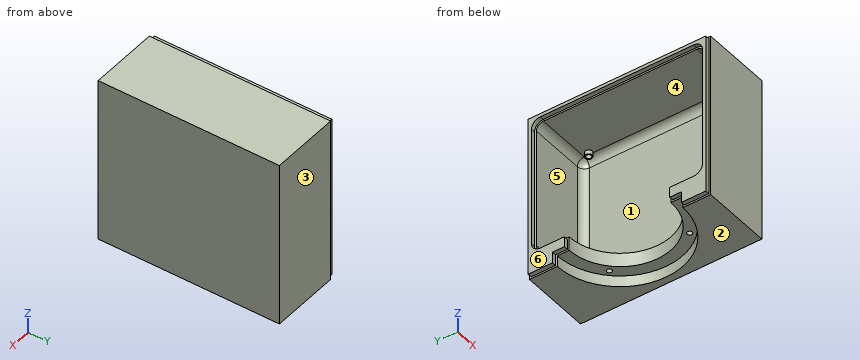
Autodesk Inventor part; units mm, degrees
ref_plane "Work Plane1" through (-95, 0, -119) normal (-1, 0, 0) x (0, 0, 1)
ref_plane "Work Plane2" through (-50, 0, -119) normal (-1, 0, 0) x (0, 0, 1)
ref_plane "YZ Plane" through (0, 0, 0) normal (1, 0, 0) x (0, 1, 0)
sketch "Sketch1" plane through (0, 0, 0) normal (0, 1, 0) x (-1, 0, 0)
  line L0 (0, 0) -> (100, 0)
  line L1 (100, 0) -> (100, -119)
  line L2 (100, -119) -> (0, -119)
  line L3 (0, -119) -> (0, 0)
  dimension "d0" = 119
  dimension "d1" = 100
extrude "Extrusion1" add sketch "Sketch1" along normal blind 130
sketch "Sketch2" plane through (0, 0, -119) normal (0, 0, -1) x (-1, 0, 0)
  circle A0 centre (50, 65) radius 45
  line L0 (100, 0) -> (100, 130)
  line L1 (0, 0) -> (0, 130)
  line L2 (0, 0) -> (100, 0)
  line L3 (0, 130) -> (100, 130)
  circle A1 centre (50, 65) radius 36.5
  circle A2 centre (28.0236, 99.1226) radius 1.9
  line L4 (25.6342, 102.8326) -> (74.3658, 27.1674) construction
  line L5 (12.1674, 40.6342) -> (87.8326, 89.3658) construction
  dimension "d6" = 90
  dimension "d7" = 100
  dimension "d8" = 50
  dimension "d9" = 65
  dimension "d10" = 130
  dimension "d11" = 73
  dimension "d12" = 3.8
extrude "Extrusion2" cut sketch "Sketch2" against normal blind 8 contours A0 | A1 | A2
extrude "Extrusion3" cut sketch "Sketch2" against normal blind 18 contours A1
ref_plane "Work Plane1" through (-95, 0, -119) normal (-1, 0, 0) x (0, 0, 1)
sketch "Sketch3" plane through (-95, 0, -119) normal (-1, 0, 0) x (0, 0, 1)
  line L0 (18, 28.5) -> (18, 101.5)
  line L1 (119, 130) -> (119, 0)
  line L2 (119, 0) -> (0, 0)
  line L3 (0, 0) -> (0, 65)
  line L4 (8, 65) -> (0, 65)
  line L5 (0, 130) -> (119, 130)
  line L6 (0, 65) -> (0, 130)
  line L7 (114, 125) -> (18, 125)
  line L8 (18, 125) -> (18, 5)
  line L9 (18, 5) -> (114, 5)
  line L10 (114, 5) -> (114, 125)
  dimension "d16" = 5
  dimension "d17" = 5
  dimension "d18" = 5
extrude "Extrusion4" cut sketch "Sketch3" against normal blind 90 and the other way blind 90 contours L0 L8 L7 L10 L9
fillet "Fillet1" radius 5 8 edges at (-52.5, 5, -5) (-5, 5, -53) (-5, 65, -5) (-5, 125, -53) (-52.5, 125, -5) (-52.5, 5, -101) (-52.5, 125, -101) (-5, 65, -101)
sketch "Sketch8" plane through (-100, 0, -119) normal (-1, 0, 0) x (0, 0, 1)
  point P0 (119, 0)
sketch "Sketch10" plane through (-100, 0, -119) normal (-1, 0, 0) x (0, 0, 1)
  line L0 (0, 0) -> (119, 0)
  line L1 (119, 0) -> (119, 130)
  line L2 (0, 130) -> (119, 130)
  line L3 (0, 0) -> (0, 130)
extrude "Extrusion10" add sketch "Sketch10" along normal blind 5
sketch "Sketch12" plane through (0, 130, 0) normal (0, 1, 0) x (1, 0, 0)
  line L0 (0, 119) -> (-105, 119)
  line L1 (-105, 0) -> (-105, 119)
  line L2 (0, 0) -> (-105, 0)
  line L3 (0, 0) -> (0, 119)
  line L4 (-105, 0) -> (-100, 0)
  line L5 (-100, 0) -> (-100, 119)
  line L6 (-100, 119) -> (-105, 119)
  line L7 (-105, 119) -> (-105, 0)
  line L8 (-100, 20) -> (-105, 25)
  line L9 (-105, 40) -> (-100, 45)
  line L10 (-105, 94) -> (-100, 99)
  line L11 (-100, 74) -> (-105, 79)
  dimension "d82" = 119
  dimension "d86" = 5
  dimension "d87" = 45
  dimension "d88" = 45
  dimension "d90" = 45
  dimension "d91" = 45
  dimension "d92" = 20
  dimension "d93" = 25
  dimension "d94" = 20
  dimension "d95" = 25
extrude "Extrusion11" cut sketch "Sketch12" against normal blind 127 contours L5 L11 L1 L10 | L8 L1 L9 L5
fillet "Fillet2" radius 1 8 edges at (-105, 66.5, -25) (-100, 127.5, -20) (-105, 66.5, -40) (-100, 127.5, -45) (-105, 66.5, -79) (-100, 127.5, -74) (-105, 66.5, -94) (-100, 127, -99)
sketch "Sketch13" plane through (-10, 120, -5) normal (0, 0, -1) x (-1, 0, 0)
  line L0 (82.5, 0) -> (-2.5, 0)
  line L1 (-2.5, 0) -> (-2.5, -110)
  line L2 (-2.5, -110) -> (82.5, -110)
  line L3 (82.5, -110) -> (82.5, 0)
  line L4 (-5, 0) -> (-5, -110)
  line L5 (85, -110) -> (85, 0)
  circle A0 centre (78.5, -4.3) radius 1.8
  circle A1 centre (78.5, -4.3) radius 2.5
  line L6 (78.5, -4.3) -> (78.5, -140.0823) construction
  line L7 (78.5, -4.3) -> (-34.9987, -4.3) construction
  line L8 (1.5, 27.6777) -> (1.5, -220.2724) construction
  line L9 (-45.8754, -105.7) -> (99.6232, -105.7) construction
  line L10 (80, 5) -> (0, 5) construction
  line L11 (0, -115) -> (80, -115) construction
  circle A2 centre (78.5, -105.7) radius 1.8
  circle A3 centre (78.5, -105.7) radius 2.5
  circle A4 centre (1.5, -105.7) radius 1.8
  circle A5 centre (1.5, -105.7) radius 2.5
  circle A6 centre (1.5, -4.3) radius 1.8
  circle A7 centre (1.5, -4.3) radius 2.5
  point P0 (-10, -120)
  dimension "d97" = 85
  dimension "d98" = 110
  dimension "d99" = 90
  dimension "d100" = 2.5
  dimension "d101" = 4
  dimension "d102" = 4.3
  dimension "d103" = 3.6
  dimension "d104" = 5
  dimension "d105" = 4.3
  dimension "d107" = 120
  dimension "d108" = 5
  dimension "d109" = 4
  dimension "d110" = 3.6
  dimension "d111" = 5
  dimension "d112" = 3.6
  dimension "d113" = 5
  dimension "d114" = 3.6
  dimension "d115" = 5
extrude "Extrusion12" add sketch "Sketch13" along normal blind 3 contours A1 | A3 | A5 | A7
sketch "Sketch14" plane through (-105, 0, -119) normal (-1, 0, 0) x (0, 0, 1)
  line L0 (19.5, 52) -> (19.5, 34) construction
  line L1 (18, 52) -> (18, 34)
  line L2 (21, 34) -> (21, 52)
  arc A0 (21, 52) -> (18, 52) centre (19.5, 52) ccw
  arc A1 (18, 34) -> (21, 34) centre (19.5, 34) ccw
  line L3 (0, 130) -> (0, 0)
  line L4 (0, 0) -> (119, 0)
  point P0 (19.5, 43)
  dimension "d118" = 18
  dimension "d119" = 3
  dimension "d121" = 18
  dimension "d122" = 34
extrude "Extrusion13" cut sketch "Sketch14" against normal blind 20
sketch "Sketch15" plane through (-50, 65, -111) normal (0, 0, -1) x (-1, 0, 0)
  circle A0 centre (0, 0) radius 45 construction
  line L0 (31.8198, 31.8198) -> (-31.8198, -31.8198) construction
  line L1 (31.8198, -31.8198) -> (-31.8198, 31.8198) construction
  circle A1 centre (0, 0) radius 36.5 construction
  circle A2 centre (0, 0) radius 40.75 construction
  line L2 (0, -45) -> (0, 45) construction
  line L3 (-40, -60) -> (40, -60) construction
  circle A3 centre (28.8146, 28.8146) radius 1.8
  circle A4 centre (-28.8146, 28.8146) radius 1.8
  circle A5 centre (28.8146, -28.8146) radius 1.8
  circle A6 centre (-28.8146, -28.8146) radius 1.8
  point P0 (-50, -65)
  dimension "d125" = 45
  dimension "d126" = 73
  dimension "d129" = 90
  dimension "d130" = 4.25
  dimension "d131" = 3.6
  dimension "d135" = 3.6
  dimension "d136" = 3.6
  dimension "d137" = 3.6
extrude "Extrusion14" cut sketch "Sketch15" against normal blind 40
ref_plane "Work Plane2" through (-50, 0, -119) normal (-1, 0, 0) x (0, 0, 1)
split "Split1" plane through (-50, 0, -119) removes the side toward (-1, 0, 0)
sketch "Sketch18" plane through (-50, 0, -119) normal (-1, 0, 0) x (0, 0, 1)
  line L0 (8, 110) -> (0, 110)
  line L1 (8, 101.5) -> (8, 110)
  line L2 (18, 101.5) -> (8, 101.5)
  line L3 (18, 120) -> (18, 101.5)
  arc A0 (23, 125) -> (18, 120) centre (23, 120) ccw
  line L4 (109, 125) -> (23, 125)
  arc A1 (114, 120) -> (109, 125) centre (109, 120) ccw
  line L5 (114, 10) -> (114, 120)
  arc A2 (109, 5) -> (114, 10) centre (109, 10) ccw
  line L6 (23, 5) -> (109, 5)
  arc A3 (18, 10) -> (23, 5) centre (23, 10) ccw
  line L7 (18, 28.5) -> (18, 10)
  line L8 (8, 28.5) -> (18, 28.5)
  line L9 (8, 20) -> (8, 28.5)
  line L10 (0, 20) -> (8, 20)
  line L11 (0, 0) -> (0, 20)
  line L12 (119, 0) -> (0, 0)
  line L13 (119, 130) -> (119, 0)
  line L14 (0, 130) -> (119, 130)
  line L15 (0, 110) -> (0, 130)
  line L16 (117.7, 1.3) -> (1.3, 1.3)
  line L17 (1.3, 1.3) -> (1.3, 18.7)
  line L18 (1.3, 18.7) -> (9.3, 18.7)
  line L19 (9.3, 18.7) -> (9.3, 27.2)
  line L20 (9.3, 27.2) -> (16.7, 27.2)
  line L21 (16.7, 27.2) -> (16.7, 10)
  arc A4 (16.7, 10) -> (23, 3.7) centre (23, 10) ccw
  line L22 (23, 3.7) -> (109, 3.7)
  arc A5 (109, 3.7) -> (115.3, 10) centre (109, 10) ccw
  line L23 (115.3, 10) -> (115.3, 120)
  arc A6 (115.3, 120) -> (109, 126.3) centre (109, 120) ccw
  line L24 (109, 126.3) -> (23, 126.3)
  arc A7 (23, 126.3) -> (16.7, 120) centre (23, 120) ccw
  line L25 (16.7, 120) -> (16.7, 102.8)
  line L26 (16.7, 102.8) -> (9.3, 102.8)
  line L27 (9.3, 102.8) -> (9.3, 111.3)
  line L28 (9.3, 111.3) -> (1.3, 111.3)
  line L29 (1.3, 111.3) -> (1.3, 128.7)
  line L30 (1.3, 128.7) -> (117.7, 128.7)
  line L31 (117.7, 128.7) -> (117.7, 1.3)
  dimension "d140" = 1.3
extrude "Extrusion15" add sketch "Sketch18" along normal blind 3 contours L16 L17 L18 L19 L20 L21 A4 L22 A5 L23 A6 L24 A7 L25 L26 L27 L28 L29 L30 L31
equation "\"d8\" = 0.5 * d7"
equation "\"d9\" = 0.5 * d10"
equation "\"d100\" = -0.5 * d97 + 0.5 * d99"
equation "\"d108\" = -0.5 * d98 + 0.5 * d107"
equation "\"d130\" = -0.25 * d126 + 0.25 * d129"
equation "\"d135\" = d131"
equation "\"d136\" = d131"
equation "\"d137\" = d131"
properties part number "wooferBoxTongue"
Source: CAD feature listing. Evaluate the final solid. Frame: model axes, mm. Face numbers are marked on the shaded views. A direction names the side the tool comes from. Coordinates: 2 decimals unless noted, no trailing zeros. Loops run counter-clockwise (first coordinate to the right, second up) from the corner with the lowest first, then second, coordinate; pieces in that order, holes last. Notation, with made-up numbers: M -8,-5.75 L 5,-5.75 A10 ccw 5,2.25 Z; hole C 54,24.5 d1. An arc over 180 degrees is marked long. Put each result on its own line as item: value. Start each with the question number.
1) Cut plane A-A on y = 65. Return the cut outline in (x, z).
2) Cut plane D-D on x = -39. Return the cut outline in (y, z).
3) Pull-direction query (Z, two-part tool) for the marked faces 1, 2, 3 and 4; classes: pulls with the +Z half, pulls with the -Z half, needs draft (parallel to the pull), parting line crosses it, or undercut.
4) Reachability of the marked faces 5 and 6 from +Z, -Z, +X, -X, +Y, -Y: full face, straight path, thin tool, end or side. Return the list, or none.
5) Ray query, L1, parallel to Y at x = -46, z = -41.5; L2, parallel to X at y = 14.3, z = -6.45; L3, parallel to Z at x = -27, y = 29. Return the intervals inside material, ascending. Write a range as from..to.
6) Cut plane B-B on z = -65. Return the cut outline in (x, y).
7) Contact query for flat-ended pins moving along their axis: pin 1 Ø0.9 at (x, z) = (-51, -113) entering from +Y; pin 2 Ø1 at (x, y) = (-11.5, 85) entering from -Z; pin 3 Ø10 at (y, z) = (67.5, -97.5) entering from -X; pin 4 Ø1.5 at (x, z) = (-31, -22) entering from -Y. Output: stop coordinate, or through.
The answers:
1. outline: M -53,-3.7 L -50,-3.7 L -50,-5 L -10,-5 A5 cw -5,-10 L -5,-96 A5 cw -10,-101 L -13.5,-101 L -13.5,-111 L -5,-111 L -5,-119 L 0,-119 L 0,0 L -50,0 L -50,-1.3 L -53,-1.3 Z
2. outline: M 0,-119 L 21.37,-119 L 21.37,-111 L 30.2,-111 L 30.2,-101 L 10,-101 A5 cw 5,-96 L 5,-10 A5 cw 10,-5 L 120,-5 A5 cw 125,-10 L 125,-96 A5 cw 120,-101 L 99.8,-101 L 99.8,-111 L 108.63,-111 L 108.63,-119 L 130,-119 L 130,0 L 0,0 Z
3. face 1: undercut
3. face 2: pulls with the -Z half
3. face 3: needs draft
3. face 4: undercut
4. face 5: -X
4. face 6: +Z, -Z, -X, +Y, -Y
5. L1: y = 0..5, 125..130
5. L2: x = -14..-13.3, -9.7..-9, -6.48..0
5. L3: z = -111..-101, -5..0
6. outline: M -53,1.3 L -50,1.3 L -50,0 L 0,0 L 0,130 L -50,130 L -50,128.7 L -53,128.7 L -53,126.3 L -50,126.3 L -50,125 L -10,125 A5 cw -5,120 L -5,10 A5 cw -10,5 L -50,5 L -50,3.7 L -53,3.7 Z
7. pin 1: stops at y = 128.7
7. pin 2: stops at z = -111
7. pin 3: stops at x = -14.01
7. pin 4: stops at y = 0
